CAD build for the part. Positions are in the model's coordinates, mm. A direction names the side the tool comes from. Coordinates: 2 decimals unless noted, no trailing zeros. Order: outer loops, then holes, each group sorted by start corner. A loop starts at its lowest first (then second) coordinate and runs counter-clockwise, first axis right, second up. Notation, with made-up numbers: M 71,89 L 112,89 A21 ccw 112,113 Z; hole C 76.25,29 d2. An arc over 180 degrees is marked long. Write item = value, one per line.
from build123d import *

# Parameters (mm, degrees)
EXTRUDE1_DEPTH     = 12.5
SKETCH2_W          = 50
SKETCH2_H          = 20
CUT_EXTRUDE1_DEPTH = 21
SKETCH3_R          = 3.5
EXTRUDE2_DEPTH     = 70
SKETCH4_R          = 6.25
EXTRUDE3_DEPTH     = 15
SKETCH7_R          = 6.25
SKETCH7_R_2        = 3.25
EXTRUDE6_DEPTH     = 5
SKETCH6_R          = 4
EXTRUDE5_DEPTH     = 20


with BuildPart() as part:
    # Sketch1 → Extrude1 (new body, symmetric)
    with BuildSketch(Plane.XY):
        with BuildLine():
            Line((50, 10), (0, 10))
            ThreePointArc((0, 10), (-10, 0), (0, -10))
            Line((0, -10), (50, -10))
            ThreePointArc((50, -10), (60, 0), (50, 10))
        make_face()
    extrude(amount=EXTRUDE1_DEPTH, both=True)

    # Sketch2 → Cut-Extrude1 (cut, through all)
    with BuildSketch(Plane(origin=(0, 10, 0), x_dir=(-1, 0, 0), z_dir=(0, 1, 0))):
        with Locations((-11, 0)):
            Rectangle(SKETCH2_W, SKETCH2_H)
    extrude(amount=-CUT_EXTRUDE1_DEPTH, mode=Mode.SUBTRACT)

    # Sketch3 → Extrude2 (add)
    with BuildSketch(Plane.YZ.offset(50)):
        with Locations((0, 11)):
            Circle(SKETCH3_R)
    extrude2 = extrude(amount=EXTRUDE2_DEPTH)

    # Mirror1: Extrude2 across plane
    add(extrude2.mirror(Plane.XY))

    # Sketch4 → Extrude3 (add, symmetric)
    with BuildSketch(Plane.XY):
        with Locations((125, 0)):
            Circle(SKETCH4_R)
    extrude(amount=EXTRUDE3_DEPTH, both=True)

    # Sketch7 → Extrude6 (cut, symmetric)
    with BuildSketch(Plane.XY):
        with Locations((125, 0)):
            Circle(SKETCH7_R)
        with Locations((125, 0)):
            Circle(SKETCH7_R_2, mode=Mode.SUBTRACT)
    extrude(amount=EXTRUDE6_DEPTH, both=True, mode=Mode.SUBTRACT)

    # Sketch6 → Extrude5 (add)
    with BuildSketch(Plane.XY.offset(-10)):
        Circle(SKETCH6_R)
    extrude(amount=EXTRUDE5_DEPTH)


solid = part.part
(1) Slice it at B-B, the plane y = 0. State how many separate pieces and enclosed holes the cut face has, then the cut area to 3 significant figures.
Evaluation:
separate_pieces = 1
enclosed_holes = 2
area = 2,170 mm²
(2) Wall check: line 1 (Z direction, x = 27.5, y = -5.5); line 2 (X direction, y = -1.25, z = 7.5); line 3 (Y direction, x = 117, z = -11). Give the ranges that are in metal, low to high. Write a range as from..to.
Evaluation:
line_1 = -12.5..-10, 10..12.5
line_2 = -3.8..3.8, 36..59.92, 118.88..131.12
line_3 = -3.5..3.5
(3) Pin check, flat tips, straight feed: pin 1 Ø12 at (y, z) = (-2.5, -6.5) entering from +X; pin 2 Ø1 at (x, y) = (80.5, -3) entering from +Z; pin 3 Ø2 at (y, z) = (1, 14) entering from -X; pin 4 Ø6 at (x, y) = (15, -2) entering from +Z. Stop position of each tip, or through.
Evaluation:
pin_1 = 131.25
pin_2 = 13.45
pin_3 = 50
pin_4 = 12.5
(4) Slice it at C-C, the plane z = -1. Write the cut outline in (x, y).
Evaluation:
outline = C 0,0 d8; M 36,-10 L 50,-10 A10 ccw 50,10 L 36,10 Z; C 125,0 d6.5
(5) Pull direction Z, two halves, no side cores. Call faces 4 (the face through (24, 0, -12.5)), 5 (the face through (41, -10, 0)), 6 (the face through (128, -3, -5)): +Z half, -Z half, draft (parallel to the pull), parting line (faces both ways), or undercut.
Evaluation:
face_4 = -Z half
face_5 = draft
face_6 = undercut
(6) Slice it at A-A, the plane x = 17. Write the cut outline in (y, z).
Evaluation:
outline = M -10,-12.5 L 10,-12.5 L 10,-10 L -10,-10 Z; M -10,10 L 10,10 L 10,12.5 L -10,12.5 Z
(7) Slice it at D-D, the plane y = -8. Write the cut outline in (x, z), then the cut area to 3 significant figures.
Evaluation:
outline = M -6,-12.5 L 56,-12.5 L 56,12.5 L -6,12.5 L -6,10 L 36,10 L 36,-10 L -6,-10 Z
area = 710 mm²
(8) Tool access for faces 1 (the face through (84.42, -0.46, -14.47)), 2 (the face through (-10, 0, -11)), 3 (the face through (36, 0, 0)): list every direction of +Z, -Z, +X, -X, +Y, -Y with a clear straight run to the whole face (end or side of a thin tool).
Evaluation:
face_1 = none
face_2 = +Z, -Z, -X
face_3 = +Y, -Y
